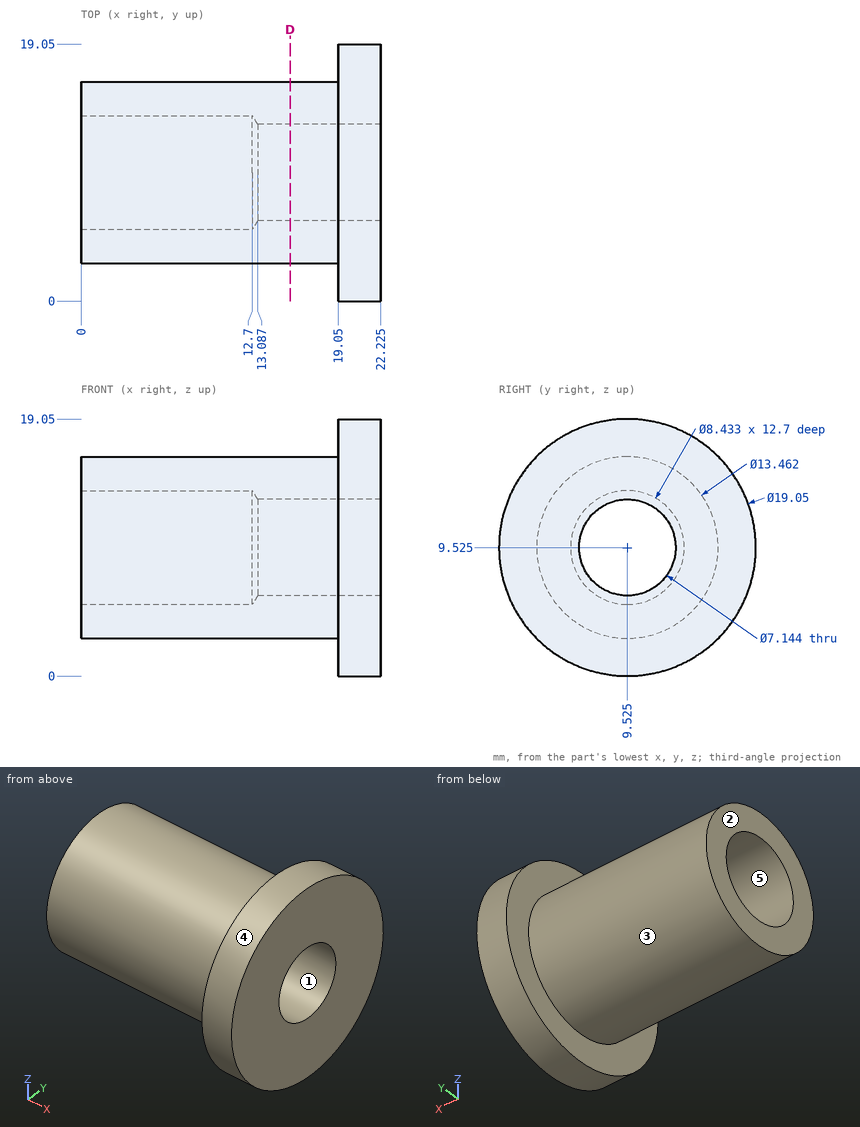
Here's the drawing with two shaded views (mm, measured from the low corner). I have some questions. A direction names the side the tool comes from. Coordinates: 2 decimals unless noted, no trailing zeros. Write each loop counter-clockwise with the first axis right and the second up, starting at its lowest first coordinate (ties: lowest second). Pieces come first, ordered by that corner, then holes. Notation, with made-up numbers: M 37,-15.75 L 79,-15.75 A30 ccw 79,9.25 Z; hole C -7.75,22 d6. An arc over 180 degrees is marked long. Write item = value, one per line. Start each with the question number.
Q1. Thinking about a two-plate mould opening in Z: for the marked faces 1, 2 and 3, which applies, released by +Z, released by -Z, zero draft, split by the parting line, or undercut?
Q2. If I drill on L1, parallel to Z at x = 13.75, y = 11.75; L2, parallel to Z at x = 5, y = 6.75; L3, parallel to Y at x = 14.5, z = 6.5 (1 decimal), over which ranges is the centre line in solid material (lowest first)? Write a range as [from, to].
Q3. I'm going to push flat-ended pins straight in: pin 1 (10 mm diameter, centred on y = 11.5, z = 6, fed in from -X); pin 2 (6 mm diameter, centred on x = 14.5, z = 3.5, fed in from -Y); pin 3 (1 mm diameter, centred on x = 7.5, y = 7.5, fed in from +Z); pin 4 (10 mm diameter, centred on x = 11, y = 11.5, fed in from -Z). Where does each tip first touch, or does it pass through?
Q4. On a 3-axis mill with a long thin cutter (end or side, diameter ignored), from which of +Z, -Z, +X, -X, +Y, -Y can I reach the whole of each face in a straight line? I mean the marked faces 4 and 5. Say none if no direction works.
Q5. If we section it at D-D, the plane x = 15.5: Write out the boundary of the cut face in (y, z) (1 decimal).
Check sheet entries:
q1.face_1 = undercut
q1.face_2 = zero draft
q1.face_3 = split by the parting line
q2.L1 = [3.17, 6.73], [12.32, 15.88]
q2.L2 = [3.39, 6.35], [12.7, 15.66]
q2.L3 = [3.5, 7.6], [11.4, 15.5]
q3.pin_1 = 0
q3.pin_2 = 3.51
q3.pin_3 = 16.08
q3.pin_4 = 2.79
q4.face_4 = +X, -X
q4.face_5 = -X
q5.outline = C 9.5,9.5 d13.5; hole C 9.5,9.5 d7.1
